Drawing for the job (mm, zero at the part's lowest x, y, z). A direction names the side the tool comes from. Coordinates: 2 decimals unless noted, no trailing zeros. Write each loop counter-clockwise with the first axis right and the second up, starting at its lowest first coordinate (ties: lowest second). Pieces come first, ordered by that corner, then holes. Notation, with made-up numbers: (-26.75, -11) -> (-8.75, -11) arc R34 ccw to (-8.75, 28) -> close; hole circle Ø3 at (59, 43.5). An arc over 180 degrees is marked (long way). Write item = value, one per line. Start each with the question number.
Q1. Pull direction Y, two halves, no side cores. Call the marked faces 4, 5, 6 and 7: released by +Y, released by -Y, zero draft, split by the parting line, or undercut.
Q2. Band-saw the part on A-A, the plane z = 10.75. List the corners of the cut face in (x, y) (1 decimal).
Q3. Pin check, flat tips, straight feed: P1, Ø5, axis at y = 12, z = 1.5, coming from the +X side (1 decimal); P2, Ø3, axis at y = 49.5, z = 12, coming from the -X side (1 decimal); P3, Ø1.7, axis at y = 59, z = 5.5, coming from the -X side; P4, Ø8, axis at x = 9, z = 8.5, coming from the -Y side. Stop position of each tip, or through.
Q4. Tool access for the marked faces 1, 2 and 3: list every direction of +Z, -Z, +X, -X, +Y, -Y with a clear straight run to the whole face (end or side of a thin tool).
Q5. Probe line 1 (Y direction, x = 24, z = 8.5) (1 decimal); line 2 (Z direction, x = 10, y = 38); line 3 (X direction, y = 40.5, z = 3.25) (1 decimal). List the from-to ranges inside material, lowest first.
Q6. Band-saw the part on B-B, the plane x = 29.5. List the corners of the cut face in (y, z) (1 decimal), plus the area to 3 significant figures.
Q7. Band-saw the part on C-C, the plane y = 46.5. List the corners of the cut face in (x, z) (1 decimal).
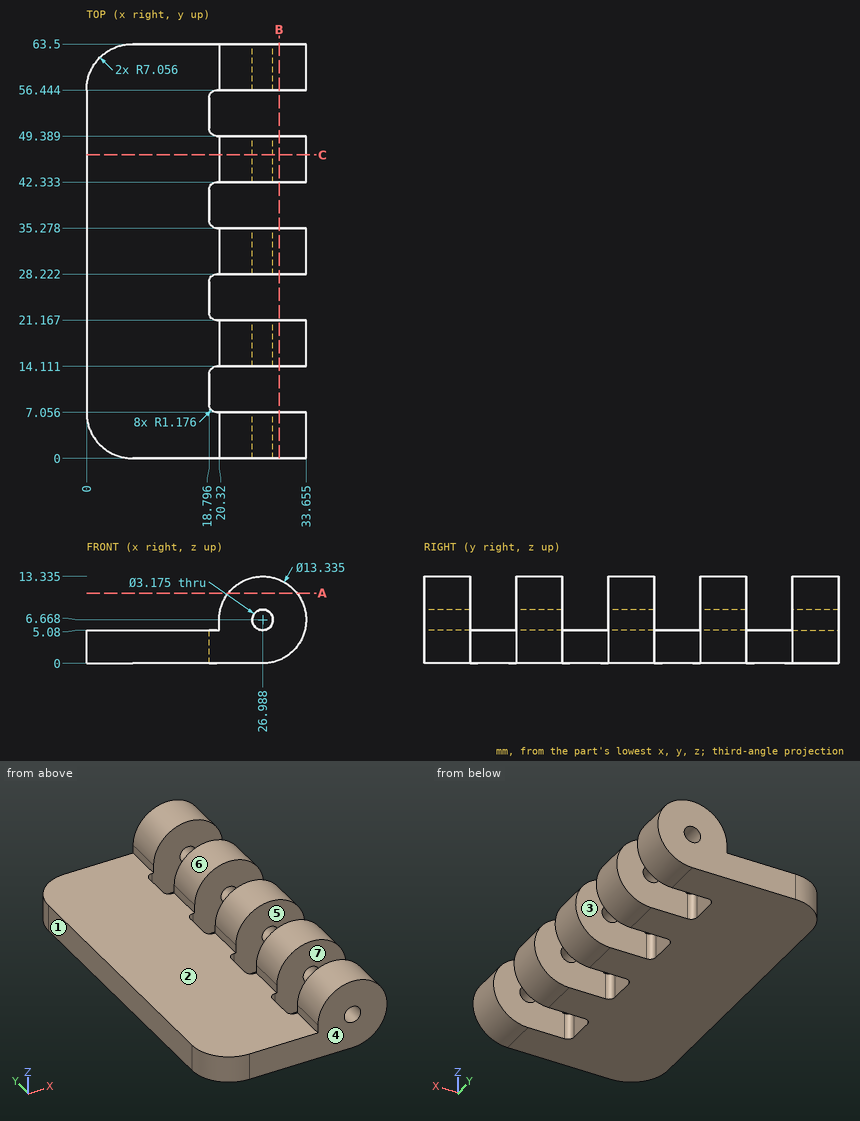
Ans:
q1.face_4 = released by -Y
q1.face_5 = undercut
q1.face_6 = zero draft
q1.face_7 = undercut
q2.outline = (21.7, 0) -> (32.3, 0) -> (32.3, 7.1) -> (21.7, 7.1) -> close; (21.7, 14.1) -> (32.3, 14.1) -> (32.3, 21.2) -> (21.7, 21.2) -> close; (21.7, 28.2) -> (32.3, 28.2) -> (32.3, 35.3) -> (21.7, 35.3) -> close; (21.7, 42.3) -> (32.3, 42.3) -> (32.3, 49.4) -> (21.7, 49.4) -> close; (21.7, 56.4) -> (32.3, 56.4) -> (32.3, 63.5) -> (21.7, 63.5) -> close
q3.P1 = 32.4
q3.P2 = 21.5
q3.P3 = 0.24
q3.P4 = 0
q4.face_1 = +Z, -Z, -X, +Y, -Y
q4.face_2 = +Z, -X, +Y, -Y
q4.face_3 = +Z, -Z, +X
q5.line_1 = 0 to 7.1, 14.1 to 21.2, 28.2 to 35.3, 42.3 to 49.4, 56.4 to 63.5
q5.line_2 = 0 to 5.08
q5.line_3 = 0 to 18.8
q6.outline = (0, 0.5) -> (7.1, 0.5) -> (7.1, 12.8) -> (0, 12.8) -> close; (14.1, 0.5) -> (21.2, 0.5) -> (21.2, 12.8) -> (14.1, 12.8) -> close; (28.2, 0.5) -> (35.3, 0.5) -> (35.3, 12.8) -> (28.2, 12.8) -> close; (42.3, 0.5) -> (49.4, 0.5) -> (49.4, 12.8) -> (42.3, 12.8) -> close; (56.4, 0.5) -> (63.5, 0.5) -> (63.5, 12.8) -> (56.4, 12.8) -> close
q6.area = 436 mm2
q7.outline = (0, 0) -> (27, 0) arc R6.7 ccw (long way) to (20.3, 6.7) -> (20.3, 5.1) -> (0, 5.1) -> close; hole circle Ø3.2 at (27, 6.7)
